Work out the finished part from the listing and answer in its coordinate system (mm). Face numbers are marked on the shaded views. A direction names the side the tool comes from. Round coordinates to 2 decimals unless told otherwise and drop trailing zeros. Loops run counter-clockwise (first coordinate to the right, second up) from the corner with the lowest first, then second, coordinate; pieces in that order, holes last.
```python
from build123d import *

# Parameters (mm, degrees)
F0_R     = 6.35
F1_DEPTH = 12.7


with BuildPart() as f1:
    # F0 (on Front) → F1 (new body)
    with BuildSketch(Plane.XZ):
        with BuildLine():
            Line((11.823206, 0.789718), (12.69937, 88.773537))
            ThreePointArc((12.69937, 88.773537), (0.287554, 76.203256), (-12.680624, 88.198734))
            Line((-12.680624, 88.198734), (-99.642679, 39.977666))
            Line((-99.642679, 39.977666), (-82.499451, -30.991102))
            Line((-82.499451, -30.991102), (11.823206, -30.991102))
            Line((11.823206, -30.991102), (11.823206, 0.789718))
        make_face()
        with BuildLine():
            Line((-69.154671, 23.427376), (-78.033982, 34.313091))
            ThreePointArc((-78.033982, 34.313091), (-77.127032, 43.247431), (-68.192691, 42.340481))
            Line((-68.192691, 42.340481), (-59.313381, 31.454767))
            ThreePointArc((-59.313381, 31.454767), (-60.220331, 22.520426), (-69.154671, 23.427376))
        make_face(mode=Mode.SUBTRACT)
        Circle(F0_R, mode=Mode.SUBTRACT)
        with BuildLine():
            ThreePointArc((-12.680624, 88.198734), (0.287554, 76.203256), (12.69937, 88.773537))
            ThreePointArc((12.69937, 88.773537), (12.699843, 88.836768), (12.7, 88.9))
            ThreePointArc((12.7, 88.9), (-0.350767, 101.595155), (-12.680624, 88.198734))
        make_face()
        with Locations((0, 88.9)):
            Circle(F0_R, mode=Mode.SUBTRACT)
    extrude(amount=F1_DEPTH)


solid = f1.part
```
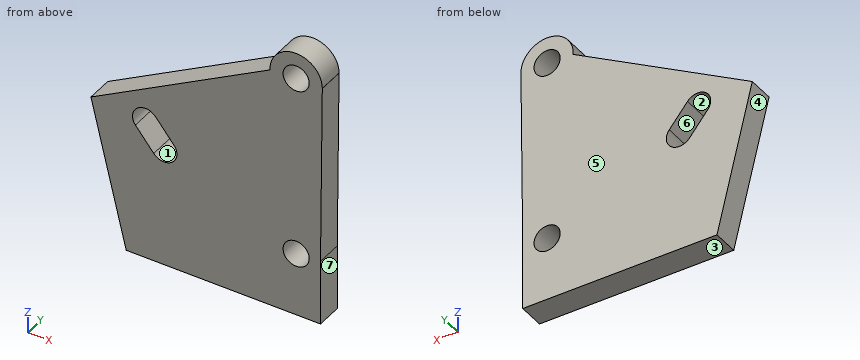
1. Consider probe 1 along Z at (x, y) = (0, -6.25); probe 2 along Z at (x, y) = (-3, -6); probe 3 along X at (y, z) = (-1, 92.5). Determine where each line is inside the solid, lowest interval first.
Answer key:
probe 1: z = -30.99 to -6.35, 6.35 to 82.55, 95.25 to 101.6
probe 2: z = -30.99 to -5.6, 5.6 to 83.3, 94.5 to 101.24
probe 3: x = -12.18 to -5.23, 5.23 to 12.18
2. Find section B-B (y = -3). Write down the section's boundary in (x, z), then the cut area to 3 significant figures.
Answer key:
outline: (-99.64, 39.98) - (-82.5, -30.99) - (11.82, -30.99) - (11.82, 0.79) - (12.7, 88.77) arc R12.65 ccw to (12.7, 88.9) arc R12.7 ccw (long way) to (-12.68, 88.2) - close; hole (-78.03, 34.31) - (-69.15, 23.43) arc R6.35 ccw to (-59.31, 31.45) - (-68.19, 42.34) arc R6.35 ccw to start; hole circle Ø12.7 at (0, 0); hole circle Ø12.7 at (0, 88.9)
area: 10,300 mm2
3. Given pin 1 (12 mm diameter, centred on x = -83, z = 8.5, fed in from +Y); pin 2 (3 mm diameter, centred on y = -5.5, z = -12, fed in from +X), each flat-ended and moving along its own axis, determine where each tip first touches the part or whether it passes through.
Answer key:
pin 1: stops at y = 0
pin 2: stops at x = 11.82
4. Determine the mould class of the marked faces 1, 2, 3 and 4 for opening direction X: +X half, -X half, draft (parallel to the pull), parting line (faces both ways), or undercut.
Answer key:
face 1: undercut
face 2: undercut
face 3: draft
face 4: -X half
5. Find section C-C (x = -27). Write down the section's boundary in (y, z).
Answer key:
outline: (-12.7, -30.99) - (0, -30.99) - (0, 80.26) - (-12.7, 80.26) - close
6. Which of the six approach directions +Z, -Z, +X, -X, +Y, -Y give full straight-line access (tool end or side, diameter ignored) to the marked faces 5, 6 and 7?
Answer key:
face 5: +Z, -Z, +X, -X, +Y
face 6: +Y, -Y
face 7: -Z, +X, +Y, -Y
7. Find section D-D (z = 53). Write down the section's boundary in (x, y), then the cut area to 3 significant figures.
Answer key:
outline: (-76.16, -12.7) - (12.34, -12.7) - (12.34, 0) - (-76.16, 0) - close
area: 1,120 mm2
8. Find section A-A (x = 0). Write down the section's boundary in (y, z).
Answer key:
outline: (-12.7, -30.99) - (0, -30.99) - (0, -6.35) - (-12.7, -6.35) - close; (-12.7, 6.35) - (0, 6.35) - (0, 82.55) - (-12.7, 82.55) - close; (-12.7, 95.25) - (0, 95.25) - (0, 101.6) - (-12.7, 101.6) - close
